from build123d import *

# Parameters (mm, degrees)
SALIENTE_EXTRUIR5_DEPTH  = 35
SALIENTE_EXTRUIR6_DEPTH  = 5
CROQUIS8_W               = 200
CROQUIS8_H               = 35
SALIENTE_EXTRUIR8_DEPTH  = 5
CROQUIS7_W               = 200
CROQUIS7_H               = 35
SALIENTE_EXTRUIR9_DEPTH  = 5
CROQUIS10_W              = 150
CROQUIS10_H              = 35
SALIENTE_EXTRUIR10_DEPTH = 5
CROQUIS11_W              = 50
CROQUIS11_H              = 17.5
CORTAR_EXTRUIR1_DEPTH    = 2.5
CROQUIS12_W              = 50
CROQUIS12_H              = 17.5
CORTAR_EXTRUIR2_DEPTH    = 2.5
CROQUIS13_W              = 55
CROQUIS13_H              = 35
SALIENTE_EXTRUIR11_DEPTH = 2.5
CROQUIS14_W              = 55
CROQUIS14_H              = 35
SALIENTE_EXTRUIR12_DEPTH = 2.5
CORTAR_EXTRUIR3_START    = -5
CORTAR_EXTRUIR3_DEPTH    = 40


with BuildPart() as part:
    # Croquis2 → Saliente-Extruir5 (new body)
    with BuildSketch(Plane(origin=(0, 0, 0), x_dir=(1, 0, 0), z_dir=(0, 1, 0))):
        with BuildLine():
            Line((-60, 70), (-120, 70))
            add(Edge.make_bspline(
                [(-120, 70), (-89.713167171, -0.733691908), (-60, 50)],
                knots=[0, 0, 0, 1, 1, 1], degree=2))
            Line((-60, 50), (0, 50))
            Line((0, 50), (0, 70))
            Line((0, 70), (-60, 70))
        make_face()
    extrude(amount=SALIENTE_EXTRUIR5_DEPTH)

    # Croquis2<6> → Saliente-Extruir6 (add)
    with BuildSketch(Plane(origin=(0, 0, 0), x_dir=(1, 0, 0), z_dir=(0, 1, 0))):
        with BuildLine():
            Line((-120, 70), (-200, 70))
            Line((-200, 70), (-200, -70))
            Line((-200, -70), (0, -70))
            Line((0, -70), (0, 50))
            Line((0, 50), (-60, 50))
            add(Edge.make_bspline(
                [(-120, 70), (-89.713167171, -0.733691908), (-60, 50)],
                knots=[0, 0, 0, 1, 1, 1], degree=2))
        make_face()
    extrude(amount=SALIENTE_EXTRUIR6_DEPTH)

    # Croquis8 → Saliente-Extruir8 (add)
    with BuildSketch(Plane(origin=(0, 0, -70), x_dir=(-1, 0, 0), z_dir=(0, 0, -1))):
        with Locations((100, 17.5)):
            Rectangle(CROQUIS8_W, CROQUIS8_H)
    extrude(amount=SALIENTE_EXTRUIR8_DEPTH)

    # Croquis7 → Saliente-Extruir9 (add)
    with BuildSketch(Plane.XY.offset(70)):
        with Locations((-100, 17.5)):
            Rectangle(CROQUIS7_W, CROQUIS7_H)
    extrude(amount=SALIENTE_EXTRUIR9_DEPTH)

    # Croquis10 → Saliente-Extruir10 (add)
    with BuildSketch(Plane.ZY.offset(200)):
        with Locations((0, 17.5)):
            Rectangle(CROQUIS10_W, CROQUIS10_H)
    extrude(amount=SALIENTE_EXTRUIR10_DEPTH)

    # Croquis11 → Cortar-Extruir1 (cut)
    with BuildSketch(Plane.XY.offset(75)):
        with Locations((-25, 17.5)):
            Rectangle(CROQUIS11_W, CROQUIS11_H)
    extrude(amount=-CORTAR_EXTRUIR1_DEPTH, mode=Mode.SUBTRACT)

    # Croquis12 → Cortar-Extruir2 (cut)
    with BuildSketch(Plane(origin=(0, 0, -75), x_dir=(-1, 0, 0), z_dir=(0, 0, -1))):
        with Locations((25, 17.5)):
            Rectangle(CROQUIS12_W, CROQUIS12_H)
    extrude(amount=-CORTAR_EXTRUIR2_DEPTH, mode=Mode.SUBTRACT)

    # Croquis13 → Saliente-Extruir11 (add)
    with BuildSketch(Plane.XY.offset(75)):
        with Locations((-27.5, 17.5)):
            Rectangle(CROQUIS13_W, CROQUIS13_H)
    extrude(amount=SALIENTE_EXTRUIR11_DEPTH)

    # Croquis14 → Saliente-Extruir12 (add)
    with BuildSketch(Plane(origin=(0, 0, -75), x_dir=(-1, 0, 0), z_dir=(0, 0, -1))):
        with Locations((27.5, 17.5)):
            Rectangle(CROQUIS14_W, CROQUIS14_H)
    extrude(amount=SALIENTE_EXTRUIR12_DEPTH)

    # Croquis15 → Cortar-Extruir3 (cut)
    with BuildSketch(Plane(origin=(0, 35, 0), x_dir=(1, 0, 0), z_dir=(0, 1, 0)).offset(CORTAR_EXTRUIR3_START)):
        with BuildLine():
            Line((-114.377865487, 70), (-5, 70))
            Line((-5, 70), (-5, 55))
            Line((-5, 55), (-62.909565923, 55))
            add(Edge.make_bspline(
                [(-62.909565923, 55), (-63.466265427, 54.021602214), (-64.401186981, 52.372327996), (-65.10401925, 51.155937563), (-66.343867423, 49.084457263), (-69.328375649, 44.517477078), (-74.11230077, 38.812847857), (-78.500104352, 35.511092249), (-81.30486337, 34.292403361), (-83.396178275, 33.823757561), (-85.433716297, 33.792096113), (-88.081814147, 34.294431754), (-92.286089613, 36.365158599), (-99.205160513, 42.585467381), (-103.799594749, 49.425151944)],
                knots=[-0.031024165, -0.031024165, -0.031024165, -0.006934179, 0.009125811, 0.025185801, 0.065335777, 0.16169572, 0.290175643, 0.386535585, 0.450775546, 0.515015508, 0.579255469, 0.675615411, 0.804095334, 0.996815219, 0.996815219, 0.996815219], degree=2))
            Line((-103.799594749, 49.425151944), (-114.377865487, 70))
        make_face()
    extrude(amount=-CORTAR_EXTRUIR3_DEPTH, mode=Mode.SUBTRACT)


solid = part.part
Verification items for the finished model (mm, model axes). A direction names the side the tool comes from. Coordinates: 2 decimals unless noted, no trailing zeros. Order: outer loops, then holes, each group sorted by start corner. A loop starts at its lowest first (then second) coordinate and runs counter-clockwise, first axis right, second up.
Item 1: Section check B-B, the plane z = -18. Enter the section's corners in (x, y), then the cut area to 4 significant figures.
Filled in:
outline: (-205, 0) - (0, 0) - (0, 5) - (-200, 5) - (-200, 35) - (-205, 35) - close
area: 1,175 mm2
Item 2: Access from +Z, -Z, +X, -X, +Y, -Y to the whole of each face (thin tool, end or side, straight path). Record for faces 1 (the face through (-159, 20, -70)), 2 (the face through (-25, 18, -75)), 3 (the face through (-5, 15, -63)).
Filled in:
face 1: +Y
face 2: +X
face 3: -Y
Item 3: Release check for a two-part mould opening along Z. For faces 4 (the face through (-205, 18, -1)), 5 (the face through (-129, 17, 75)), 6 (the face through (-25, 18, 72.5)), 7 (the face through (-25, 18, 75)) record: +Z half, -Z half, draft (parallel to the pull), parting line (faces both ways), or undercut.
Filled in:
face 4: draft
face 5: +Z half
face 6: undercut
face 7: undercut
Item 4: Material ranges on L1, parallel to Z at x = -9.5, y = 7.5; L2, parallel to Z at x = -111.5, y = 25; L3, parallel to X at y = 9.5, z = -38.5, recorded low to high.
Filled in:
L1: z = -77.5 to -70, -55 to -50, 70 to 77.5
L2: z = -75 to -70, -64.4 to -52.52, 70 to 75
L3: x = -205 to -200, -101.89 to -94.66, -74.74 to -68.05
Item 5: Section check A-A, the plane x = -13.5. Enter the section's corners in (y, z).
Filled in:
outline: (0, -77.5) - (35, -77.5) - (35, -50) - (5, -50) - (5, 70) - (35, 70) - (35, 77.5) - (0, 77.5) - (0, -55) - (30, -55) - (30, -70) - (0, -70) - close; hole (8.75, -75) - (26.25, -75) - (26.25, -72.5) - (8.75, -72.5) - close; hole (8.75, 72.5) - (26.25, 72.5) - (26.25, 75) - (8.75, 75) - close
Item 6: Section check C-C, the plane x = -129. Enter the section's corners in (y, z), then the cut area to 3 significant figures.
Filled in:
outline: (0, -75) - (35, -75) - (35, -70) - (5, -70) - (5, 70) - (35, 70) - (35, 75) - (0, 75) - close
area: 1,050 mm2
Item 7: Depth check by flat-ended pin: pin 1 (1.2 mm diameter, centred on y = 25.5, z = 76, fed in from -X); pin 2 (15 mm diameter, centred on y = 16, z = 28.5, fed in from +X); pin 3 (1 mm diameter, centred on x = -157, y = 16, fed in from +Z). Enter the tip coordinate at first touch or a pass-through.
Filled in:
pin 1: stops at x = -55
pin 2: stops at x = -200
pin 3: stops at z = 75
